The listing builds one solid part. Answer for the finished solid, in the listing's coordinates (mm). A direction names the side the tool comes from. Give positions to 0.01 mm unless a question says otherwise; leave off trailing zeros. Loops run counter-clockwise (first coordinate to the right, second up) from the corner with the lowest first, then second, coordinate; pieces in that order, holes last. Notation, with made-up numbers: M -5,-10.5 L 29,-10.5 A17 cw 29,-6.5 Z; hole C 58,55.25 d6. An arc over 180 degrees is marked long. Return JSON: item names as keys, results as strings.
from build123d import *

# Parameters (mm, degrees)
F0_W     = 19.304
F0_H     = 59.5884
F1_DEPTH = 0.762
F2_W     = 0.762
F2_H     = 59.5884
F3_DEPTH = 0.762
F4_W     = 19.304
F4_H     = 3.81
F5_DEPTH = 3.81
F6_W     = 20.828
F6_H     = 0.127
F7_DEPTH = 0.254


with BuildPart() as f1:
    # F0 (on Front) → F1 (new body)
    with BuildSketch(Plane.XZ):
        with Locations((0, 29.7942)):
            Rectangle(F0_W, F0_H)
    extrude(amount=F1_DEPTH)

    # F2 (on Front) → F3 (join)
    with BuildSketch(Plane.XZ):
        with Locations((-10.033, 29.7942)):
            Rectangle(F2_W, F2_H)
        with Locations((10.033, 29.7942)):
            Rectangle(F2_W, F2_H)
    extrude(amount=F3_DEPTH)

    # F4 (on Front) → F5 (join)
    with BuildSketch(Plane.XZ):
        with Locations((0, 61.4934)):
            Rectangle(F4_W, F4_H)
    extrude(amount=F5_DEPTH)

    # F6 (on face) → F7 (cut)
    with BuildSketch(Plane.XZ.offset(0.762)):
        with Locations((0, 1.8415)):
            Rectangle(F6_W, F6_H)
        with Locations((0, 3.6449)):
            Rectangle(F6_W, F6_H)
        with Locations((0, 5.4483)):
            Rectangle(F6_W, F6_H)
        with Locations((0, 7.2517)):
            Rectangle(F6_W, F6_H)
        with Locations((0, 9.0551)):
            Rectangle(F6_W, F6_H)
        with Locations((0, 10.8585)):
            Rectangle(F6_W, F6_H)
        with Locations((0, 12.6619)):
            Rectangle(F6_W, F6_H)
        with Locations((0, 14.4653)):
            Rectangle(F6_W, F6_H)
        with Locations((0, 16.2687)):
            Rectangle(F6_W, F6_H)
        with Locations((0, 18.0721)):
            Rectangle(F6_W, F6_H)
        with Locations((0, 19.8755)):
            Rectangle(F6_W, F6_H)
        with Locations((0, 21.6789)):
            Rectangle(F6_W, F6_H)
        with Locations((0, 23.4823)):
            Rectangle(F6_W, F6_H)
        with Locations((0, 25.2857)):
            Rectangle(F6_W, F6_H)
        with Locations((0, 27.0891)):
            Rectangle(F6_W, F6_H)
        with Locations((0, 28.8925)):
            Rectangle(F6_W, F6_H)
        with Locations((0, 30.6959)):
            Rectangle(F6_W, F6_H)
        with Locations((0, 32.4993)):
            Rectangle(F6_W, F6_H)
        with Locations((0, 34.3027)):
            Rectangle(F6_W, F6_H)
        with Locations((0, 36.1061)):
            Rectangle(F6_W, F6_H)
        with Locations((0, 37.9095)):
            Rectangle(F6_W, F6_H)
        with Locations((0, 39.7129)):
            Rectangle(F6_W, F6_H)
        with Locations((0, 41.5163)):
            Rectangle(F6_W, F6_H)
        with Locations((0, 43.3197)):
            Rectangle(F6_W, F6_H)
        with Locations((0, 45.1231)):
            Rectangle(F6_W, F6_H)
        with Locations((0, 46.9265)):
            Rectangle(F6_W, F6_H)
        with Locations((0, 48.7299)):
            Rectangle(F6_W, F6_H)
        with Locations((0, 50.5333)):
            Rectangle(F6_W, F6_H)
        with Locations((0, 52.3367)):
            Rectangle(F6_W, F6_H)
        with Locations((0, 54.1401)):
            Rectangle(F6_W, F6_H)
        with Locations((0, 55.9435)):
            Rectangle(F6_W, F6_H)
        with Locations((0, 57.7469)):
            Rectangle(F6_W, F6_H)
    extrude(amount=-F7_DEPTH, mode=Mode.SUBTRACT)


solid = f1.part
(1) A tool of negligible diameter and unlimited length cuts with its end or side. For faces 1 (the flat face through (-9.652, -2, 61)), 2 (the flat face through (9.652, -2, 61)), 3 (the flat face through (0, -0.762, 35)), from which of +Z, -Z, +X, -X, +Y, -Y can it reach the whole face along a straight path? Write none if from no direction.
Values follow:
{"face 1": "+Z, -X, +Y, -Y", "face 2": "+Z, +X, +Y, -Y", "face 3": "-Z, +X, -X, -Y"}
(2) Straight lines are drawn through the part: line 1 along Y through (x, z) = (4, 10); line 2 along Z through (x, y) = (3.75, -2.2). For each, find the intervals that lie inside material, in ascending order.
Values follow:
{"line 1": "-0.76 to 0", "line 2": "59.59 to 63.4"}
(3) Given pin 1 (1.8 mm diameter, centred on x = 1.5, z = 37.5, fed in from -Y); pin 2 (1.5 mm diameter, centred on x = 0, y = -2.5, fed in from -Z), each flat-ended and moving along its own axis, determine where each tip first touches the part or whether it passes through.
Values follow:
{"pin 1": "y = -0.76", "pin 2": "z = 59.59"}
(4) The part is cut by section B-B (z = 42.5). Determine the outline of the cut face in (x, y), and give its area (3 significant figures).
Values follow:
{"outline": "M -10.41,-0.76 L 10.41,-0.76 L 10.41,0 L -10.41,0 Z", "area": "15.9 mm²"}
(5) The part is cut by section A-A (y = -2.6). Determine the outline of the cut face in (x, z), and give its area (3 significant figures).
Values follow:
{"outline": "M -9.65,59.59 L 9.65,59.59 L 9.65,63.4 L -9.65,63.4 Z", "area": "73.5 mm²"}
